Study the drawing (mm; zero at the part's minimum x, y, z) and answer. A direction names the side the tool comes from. Round coordinates to 2 decimals unless told otherwise and drop trailing zeros. Write each loop counter-clockwise with the first axis right and the second up, starting at its lowest first coordinate (ties: lowest second). Pieces come first, ordered by that corner, then holes.
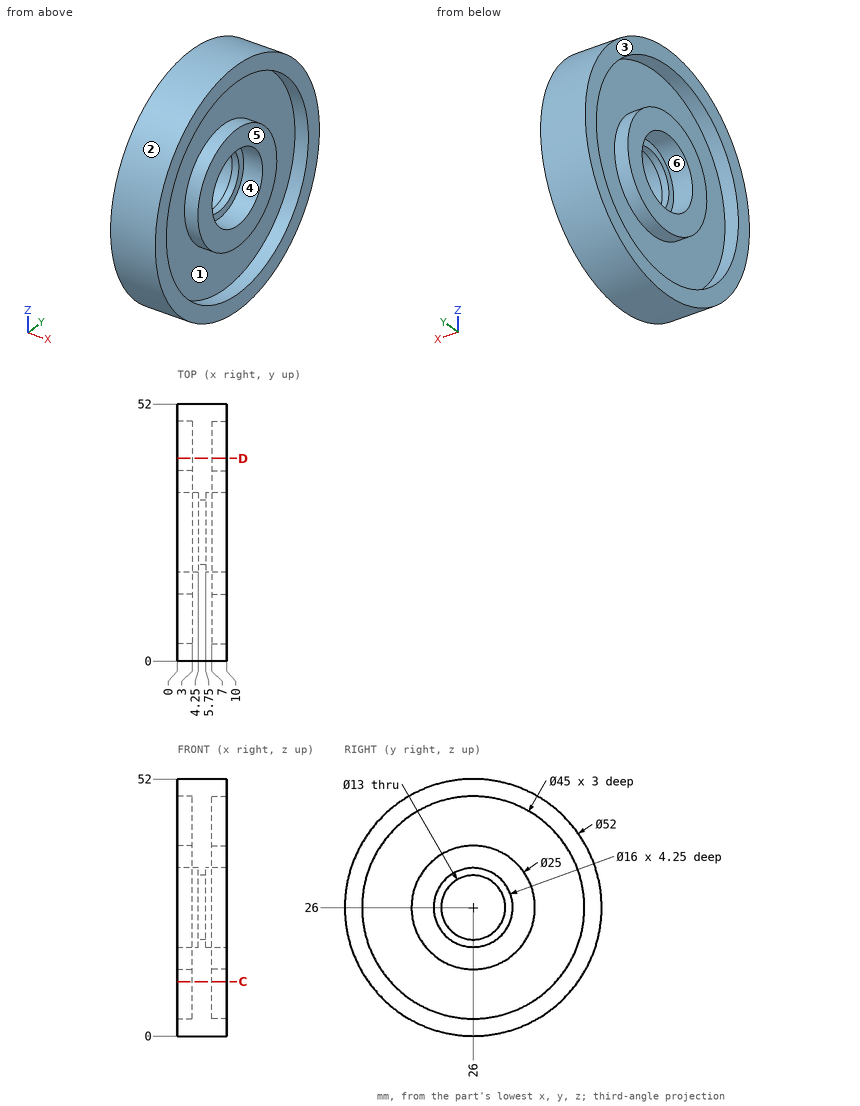
1. Section C-C on z = 11 is taken. Determine the outline of the cut face in (x, y), plus the area to 3 significant figures.
Geometry says:
outline: (0, 4.76) - (10, 4.76) - (10, 9.23) - (7, 9.23) - (7, 42.77) - (10, 42.77) - (10, 47.24) - (0, 47.24) - (0, 42.77) - (3, 42.77) - (3, 9.23) - (0, 9.23) - close
area: 223 mm2
2. Straight lines are drawn through the part: line 1 along Y through (x, z) = (1.5, 26); line 2 along Y through (x, z) = (5.05, 26); line 3 along Y through (x, z) = (9.75, 24). For each, find the intervals that lie inside material, in ascending order.
Geometry says:
line 1: y = 0 to 3.5, 13.5 to 18, 34 to 38.5, 48.5 to 52
line 2: y = 0 to 19.5, 32.5 to 52
line 3: y = 0.08 to 3.59, 13.66 to 18.25, 33.75 to 38.34, 48.41 to 51.92
3. Given pin 1 (5 mm diameter, centred on x = 3, z = 8, fed in from +Y); pin 2 (4 mm diameter, centred on x = 1.5, y = 10.5, fed in from +Z); pin 3 (2 mm diameter, centred on x = 2, z = 40.5, fed in from +Y), each flat-ended and moving along its own axis, determine where each tip first touches the part or whether it passes through.
Geometry says:
pin 1: stops at y = 46.87
pin 2: stops at z = 48.22
pin 3: stops at y = 48.22
4. A tool of negligible diameter and unlimited length cuts with its end or side. For the marked faces 4, 5 and 6, from which of +Z, -Z, +X, -X, +Y, -Y can it reach the whole face along a straight path? Write none if from no direction.
Geometry says:
face 4: +X
face 5: +Z, -Z, +X, +Y, -Y
face 6: -X
5. For a pull along Z with two mould halves and no side action, classify the marked faces 1, 2 and 3 as released by +Z, released by -Z, zero draft, split by the parting line, or undercut.
Geometry says:
face 1: undercut
face 2: split by the parting line
face 3: zero draft
